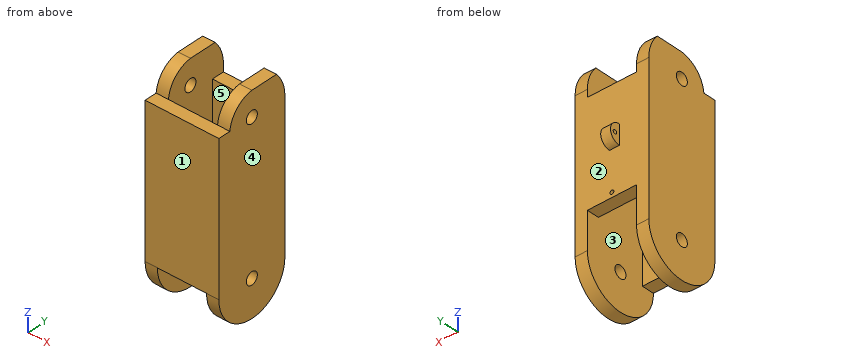
```python
from build123d import *

# Parameters (mm, degrees)
SKETCH1_W           = 19.05
SKETCH1_H           = 57.15
BOSS_EXTRUDE1_DEPTH = 19.05
SKETCH2_W           = 12.7
SKETCH2_H           = 12.7
CUT_EXTRUDE1_DEPTH  = 76.2
SKETCH3_W           = 2.54
SKETCH3_H           = 5.08
BOSS_EXTRUDE2_DEPTH = 2.54
SKETCH4_R           = 0.508
SKETCH4_R_2         = 1.5875
CUT_EXTRUDE2_DEPTH  = 19.05
SKETCH7_R           = 0.508
CUT_EXTRUDE3_DEPTH  = 12.7
SKETCH8_W           = 12.7
SKETCH8_H           = 9.525
CUT_EXTRUDE4_DEPTH  = 25.4
SKETCH11_R          = 1.5875
CUT_EXTRUDE6_DEPTH  = 19.05
SKETCH12_W          = 12.7
SKETCH12_H          = 30.970960978
CUT_EXTRUDE7_DEPTH  = 3.81
SKETCH13_W          = 12.7
SKETCH13_H          = 19.463069007
CUT_EXTRUDE8_DEPTH  = 3.81
CUT_EXTRUDE9_DEPTH  = 19.05


with BuildPart() as part:
    # Sketch1 → Boss-Extrude1 (new body)
    with BuildSketch(Plane(origin=(0, 0, 0), x_dir=(1, 0, 0), z_dir=(0, 1, 0))):
        with Locations((9.525, 28.575)):
            Rectangle(SKETCH1_W, SKETCH1_H)
    extrude(amount=BOSS_EXTRUDE1_DEPTH)

    # Sketch2 → Cut-Extrude1 (cut)
    with BuildSketch(Plane.XY):
        with Locations((9.525, 9.525)):
            Rectangle(SKETCH2_W, SKETCH2_H)
    extrude(amount=-CUT_EXTRUDE1_DEPTH, mode=Mode.SUBTRACT)

    # Sketch3 → Boss-Extrude2 (add)
    with BuildSketch(Plane(origin=(0, 19.05, 0), x_dir=(1, 0, 0), z_dir=(0, 1, 0))):
        with Locations((8.89, 24.13)):
            Rectangle(SKETCH3_W, SKETCH3_H)
    extrude(amount=BOSS_EXTRUDE2_DEPTH)

    # Sketch4 → Cut-Extrude2 (cut)
    with BuildSketch(Plane(origin=(0, 0, 0), x_dir=(0, 0, -1), z_dir=(1, 0, 0))):
        with Locations((24.13, 20.32)):
            Circle(SKETCH4_R)
        with Locations((9.525, 9.525)):
            Circle(SKETCH4_R_2)
        with BuildLine():
            ThreePointArc((26.67, 19.05), (24.13, 24.78976855), (21.59, 19.05))
            add(Edge.make_bspline(
                [(26.67, 19.05), (26.67, 21.59), (24.13, 21.59), (21.59, 21.59), (21.59, 19.05)],
                knots=[3.141592654, 3.141592654, 3.141592654, 4.71238898, 4.71238898, 6.283185307, 6.283185307, 6.283185307], degree=2, weights=[1, 0.707106781, 1, 0.707106781, 1]))
        make_face()
        with BuildLine():
            ThreePointArc((9.525, 19.05), (0, 9.525), (9.525, 0))
            ThreePointArc((9.525, 0), (-29.420443119, 9.525), (9.525, 19.05))
        make_face()
    extrude(amount=CUT_EXTRUDE2_DEPTH, mode=Mode.SUBTRACT)

    # Sketch7 → Cut-Extrude3 (cut)
    with BuildSketch(Plane(origin=(0, 19.05, 0), x_dir=(1, 0, 0), z_dir=(0, 1, 0))):
        with Locations((9.525, 36.83)):
            Circle(SKETCH7_R)
        Polygon((3.175, 0), (3.175, 11.43), (6.35, 11.43), (12.7, 11.43), (15.875, 11.43), (15.875, 0), align=None)
    extrude(amount=-CUT_EXTRUDE3_DEPTH, mode=Mode.SUBTRACT)

    # Sketch8 → Cut-Extrude4 (cut)
    with BuildSketch(Plane(origin=(0, 19.05, 0), x_dir=(1, 0, 0), z_dir=(0, 1, 0))):
        with Locations((9.525, 4.7625)):
            Rectangle(SKETCH8_W, SKETCH8_H)
    extrude(amount=-CUT_EXTRUDE4_DEPTH, mode=Mode.SUBTRACT)

    # Sketch11 → Cut-Extrude6 (cut)
    with BuildSketch(Plane(origin=(0, 0, 0), x_dir=(0, 0, -1), z_dir=(1, 0, 0))):
        with Locations((47.625, 9.525)):
            Circle(SKETCH11_R)
        with BuildLine():
            ThreePointArc((47.625, 0), (57.15, 9.525), (47.625, 19.05))
            ThreePointArc((47.625, 19.05), (63.905355935, 9.525), (47.625, 0))
        make_face()
    extrude(amount=CUT_EXTRUDE6_DEPTH, mode=Mode.SUBTRACT)

    # Sketch12 → Cut-Extrude7 (cut)
    with BuildSketch(Plane(origin=(0, 19.05, 0), x_dir=(1, 0, 0), z_dir=(0, 1, 0))):
        with Locations((9.525, 53.585480489)):
            Rectangle(SKETCH12_W, SKETCH12_H)
    extrude(amount=-CUT_EXTRUDE7_DEPTH, mode=Mode.SUBTRACT)

    # Sketch13 → Cut-Extrude8 (cut)
    with BuildSketch(Plane(origin=(0, 0, 0), x_dir=(1, 0, 0), z_dir=(0, 1, 0))):
        with Locations((9.525, 57.356534504)):
            Rectangle(SKETCH13_W, SKETCH13_H)
    extrude(amount=CUT_EXTRUDE8_DEPTH, mode=Mode.SUBTRACT)

    # Sketch14 → Cut-Extrude9 (cut)
    with BuildSketch(Plane(origin=(0, 0, 0), x_dir=(0, 0, -1), z_dir=(1, 0, 0))):
        with BuildLine():
            Line((9.525, 0), (9.525, 3.175))
            ThreePointArc((9.525, 3.175), (5.21507822, 5.21507822), (3.175, 9.525))
            Line((3.175, 9.525), (3.175, 18.741336737))
            Line((3.175, 18.741336737), (-3.728591213, 9.978700773))
            Line((-3.728591213, 9.978700773), (-2.544461104, 0))
            Line((-2.544461104, 0), (9.525, 0))
        make_face()
    extrude(amount=CUT_EXTRUDE9_DEPTH, mode=Mode.SUBTRACT)


solid = part.part
```
Geometry check sheet. Reference: the model listing, model coordinates, mm. Face numbers are marked on the shaded views. A direction names the side the tool comes from. Give positions to 0.01 mm unless a question says otherwise; leave off trailing zeros. Order: outer loops, then holes, each group sorted by start corner. A loop starts at its lowest first (then second) coordinate and runs counter-clockwise, first axis right, second up. Notation, with made-up numbers: (27, 46.5) -> (65, 46.5) arc R11 cw to (65, 54.5) -> close; hole circle Ø4 at (31, 62). An arc over 180 degrees is marked (long way). Write each question's results on one line, items separated by ' | '. Start each with the question number.
(1) Sectioned sample at A-A (y = 5.5). Enter the section's corners in (x, z) (3 decimals).
(2) Sectioned sample at C-C (z = -24.13). Give the number of separate pieces and of enclosed holes in the cut face, plus the area to 3 significant figures.
(3) Mould release check, pull along Y, two halves, no side actions. Record for the marked faces 1, 2 and 3: pulls with the +Y half, pulls with the -Y half, needs draft (parallel to the pull), parting line crosses it, or undercut.
(4) Gauge pin test, flat ends, axial feed: P1, Ø5, axis at x = 10.5, z = -39.5, coming from the +Y side; P2, Ø1, axis at x = 8.5, y = 2.5, coming from the +Z side (3 decimals); P3, Ø3, axis at y = 21, z = -25, coming from the -X side. Record the tip position at first contact, or that the pin passes through.
(5) Sectioned sample at B-B (x = 11.5). Enter the section's corners in (y, z) (3 decimals).
(6) Scan lines: line 1 (Y direction, x = 8.8, z = -24.13) (3 decimals); line 2 (X direction, y = 12.75, z = -26) (3 decimals). Record each from-to range of solid material in increasing order.
(7) Sectioned sample at D-D (z = -36.83). Enter the section's corners in (x, y) (3 decimals).
(8) Access from +Z, -Z, +X, -X, +Y, -Y to the whole of each face (thin tool, end or side, straight path). Record for the marked faces 4 and 5.
Answer below:
1) outline: (0, -56.258) -> (3.175, -56.258) -> (3.175, -4.946) -> (0, -4.946) -> close; (15.875, -56.258) -> (19.05, -56.258) -> (19.05, -4.946) -> (15.875, -4.946) -> close
2) separate pieces: 2 | enclosed holes: 1 | area: 205 mm2
3) face 1: pulls with the -Y half | face 2: pulls with the +Y half | face 3: undercut
4) P1: y = 19.05 | P2: z = -9.525 | P3: x = 7.62
5) outline: (0, -47.625) -> (3.175, -47.625) -> (3.175, -9.525) -> (0, -9.525) -> close; (15.875, -38.1) -> (19.05, -38.1) -> (19.05, -11.43) -> (15.875, -11.43) -> close
6) line 1: 0 to 3.175, 15.875 to 19.812, 20.828 to 21.59 | line 2: 0 to 3.175, 15.875 to 19.05
7) outline: (0, 0) -> (19.05, 0) -> (19.05, 19.05) -> (10.033, 19.05) -> (10.033, 15.875) -> (15.875, 15.875) -> (15.875, 3.175) -> (3.175, 3.175) -> (3.175, 15.875) -> (9.017, 15.875) -> (9.017, 19.05) -> (0, 19.05) -> close
8) face 4: +Z, -Z, +X, +Y, -Y | face 5: +Z, -Z
